Print and shaded views of the part. All mm, measured from the part's lowest x, y and z. A direction names the side the tool comes from. Round coordinates to 2 decimals unless told otherwise and drop trailing zeros. Order: outer loops, then holes, each group sorted by start corner. A loop starts at its lowest first (then second) coordinate and runs counter-clockwise, first axis right, second up.
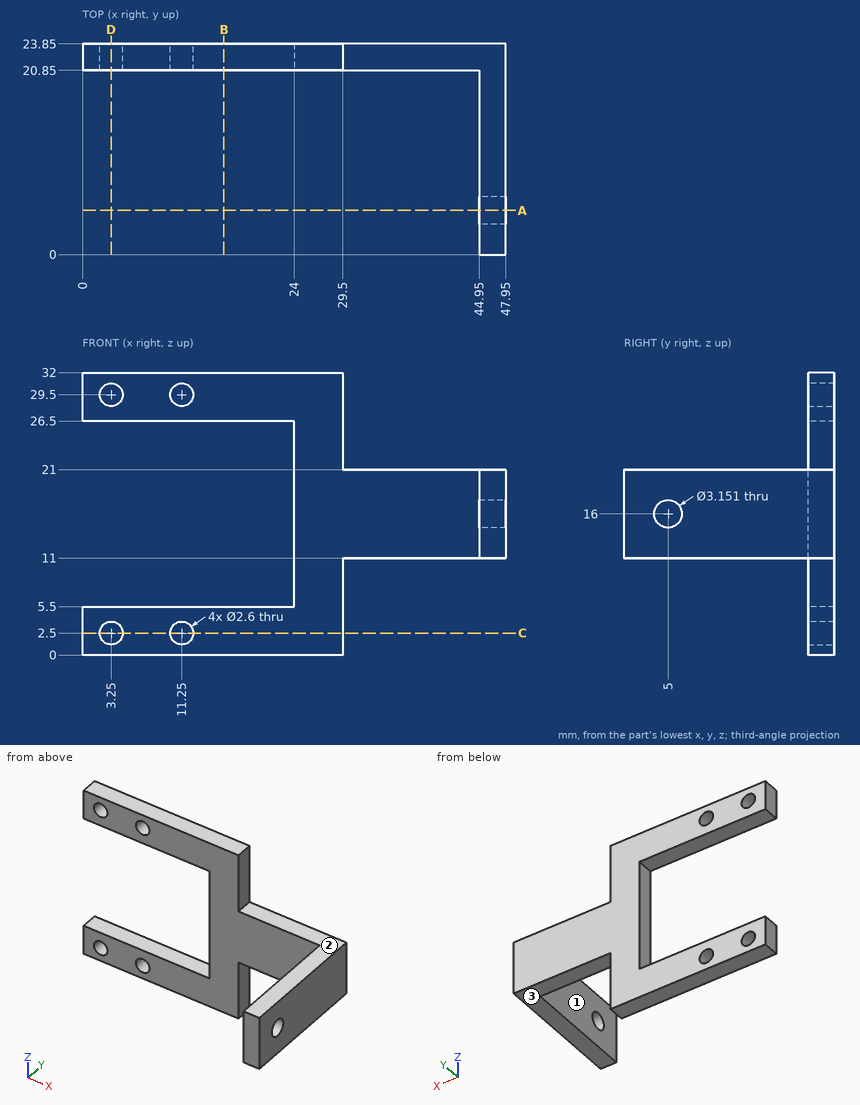
1. Drill centre lines: line 1 (X direction, y = 22.2, z = 2.5); line 2 (Y direction, x = 45.9, z = 16); line 3 (X direction, y = 6.75, z = 19). Where is each one in solid material? Low to high.
2. Cut at C-C, the plane z = 2.5. Write the cut outline in (x, y).
3. Tool access for the marked faces 1, 2 and 3: list every direction of +Z, -Z, +X, -X, +Y, -Y with a clear straight run to the whole face (end or side of a thin tool).
4. Cut at A-A, the plane y = 5. Write the cut outline in (x, z).
5. Pin check, flat tips, straight feed: P1, Ø3.5, axis at y = 22, z = 3.5, coming from the +X side; P2, Ø3.5, axis at y = 21.5, z = 11, coming from the -X side; P3, Ø4, axis at x = 11.25, z = 29.5, coming from the -Y side. Stop position of each tip, or through.
6. Cut at B-B, the plane x = 16. Write the cut outline in (y, z).
7. Cut at D-D, the plane x = 3.25. Write the cut outline in (y, z).
Outcome:
1. line 1: x = 0 to 1.95, 4.55 to 9.95, 12.55 to 29.5
1. line 2: y = 0 to 3.42, 6.58 to 23.85
1. line 3: x = 44.95 to 47.95
2. outline: (0, 20.85) - (1.95, 20.85) - (1.95, 23.85) - (0, 23.85) - close; (4.55, 20.85) - (9.95, 20.85) - (9.95, 23.85) - (4.55, 23.85) - close; (12.55, 20.85) - (29.5, 20.85) - (29.5, 23.85) - (12.55, 23.85) - close
3. face 1: +Z, -Z, -X, -Y
3. face 2: +Z, +X, +Y, -Y
3. face 3: -Z, +X, +Y, -Y
4. outline: (44.95, 11) - (47.95, 11) - (47.95, 14.42) - (44.95, 14.42) - close; (44.95, 17.58) - (47.95, 17.58) - (47.95, 21) - (44.95, 21) - close
5. P1: stops at x = 29.5
5. P2: stops at x = 24
5. P3: stops at y = 20.85
6. outline: (20.85, 0) - (23.85, 0) - (23.85, 5.5) - (20.85, 5.5) - close; (20.85, 26.5) - (23.85, 26.5) - (23.85, 32) - (20.85, 32) - close
7. outline: (20.85, 0) - (23.85, 0) - (23.85, 1.2) - (20.85, 1.2) - close; (20.85, 3.8) - (23.85, 3.8) - (23.85, 5.5) - (20.85, 5.5) - close; (20.85, 26.5) - (23.85, 26.5) - (23.85, 28.2) - (20.85, 28.2) - close; (20.85, 30.8) - (23.85, 30.8) - (23.85, 32) - (20.85, 32) - close
